from build123d import *

# Parameters (mm, degrees)
BOSS_EXTRUDE1_DEPTH  = 10
BOSS_EXTRUDE2_DEPTH  = 26.5
BOSS_EXTRUDE3_DEPTH  = 10
BOSS_EXTRUDE4_DEPTH  = 26.5
BOSS_EXTRUDE5_DEPTH  = 10
M2_CLEARANCE_HOLE1_D = 2.4


with BuildPart() as part:
    # Sketch2 → Boss-Extrude1 (new body)
    with BuildSketch(Plane.XY):
        Polygon((0, 0), (8, 0), (8, 1), (1, 1), (1, 6), (2.7, 6), (1.5, 7.2), (1, 7.2), (1, 9), (5.9, 9), (5.9, 10), (0, 10), align=None)
    extrude(amount=BOSS_EXTRUDE1_DEPTH)

    # Sketch6 → Boss-Extrude2 (add)
    with BuildSketch(Plane.XY.offset(10)):
        Polygon((0, 0), (5.9, 0), (5.9, 1), (1, 1), (1, 2.8), (2.7, 2.8), (2.7, 6), (1.5, 7.2), (1, 7.2), (1, 9), (5.9, 9), (5.9, 10), (0, 10), align=None)
    extrude(amount=BOSS_EXTRUDE2_DEPTH)

    # Sketch8 → Boss-Extrude3 (add)
    with BuildSketch(Plane.XY.offset(36.5)):
        Polygon((0, 0), (8, 0), (8, 1), (1, 1), (1, 6), (2.7, 6), (1.5, 7.2), (1, 7.2), (1, 9), (5.9, 9), (5.9, 10), (0, 10), align=None)
    extrude(amount=BOSS_EXTRUDE3_DEPTH)

    # Sketch9 → Boss-Extrude4 (add)
    with BuildSketch(Plane.XY.offset(46.5)):
        Polygon((0, 0), (5.9, 0), (5.9, 1), (1, 1), (1, 2.8), (2.7, 2.8), (2.7, 6), (1.5, 7.2), (1, 7.2), (1, 9), (5.9, 9), (5.9, 10), (0, 10), align=None)
    extrude(amount=BOSS_EXTRUDE4_DEPTH)

    # Sketch10 → Boss-Extrude5 (add)
    with BuildSketch(Plane.XY.offset(73)):
        Polygon((0, 0), (8, 0), (8, 1), (1, 1), (1, 6), (2.7, 6), (1.5, 7.2), (1, 7.2), (1, 9), (5.9, 9), (5.9, 10), (0, 10), align=None)
    extrude(amount=BOSS_EXTRUDE5_DEPTH)

    # M2 Clearance Hole1 (through all)
    with Locations(Plane(origin=(1, 0, 0), x_dir=(0, 0, -1), z_dir=(1, 0, 0))):
        with Locations((-2.8, 3.5), (-7.2, 3.5), (-39.3, 3.5), (-43.7, 3.5), (-75.8, 3.5), (-80.2, 3.5)):
            Hole(M2_CLEARANCE_HOLE1_D / 2)


solid = part.part
The model under review builds one solid part; all positions refer to its coordinate system, in mm. A direction names the side the tool comes from. Coordinates: 2 decimals unless noted, no trailing zeros. Order: outer loops, then holes, each group sorted by start corner. A loop starts at its lowest first (then second) coordinate and runs counter-clockwise, first axis right, second up. Notation, with made-up numbers: (47.5, 69) -> (100.5, 69) arc R12 cw to (100.5, 79) -> close; hole circle Ø3 at (69.5, -28.5). An arc over 180 degrees is marked (long way). Answer in a Markdown table with one row per item.
(1) Consider section A-A (x = 3.75). Write out the cut boundary in (y, z), plus the area to 3 significant figures.
Answers:
| item | result |
|---|---|
| outline | (0, 0) -> (1, 0) -> (1, 83) -> (0, 83) -> close; (9, 0) -> (10, 0) -> (10, 83) -> (9, 83) -> close |
| area | 166 mm² |
(2) Consider section B-B (z = 39.3). Write out the cut boundary in (x, y), plus the area to 3 significant figures.
Answers:
| item | result |
|---|---|
| outline | (0, 0) -> (8, 0) -> (8, 1) -> (1, 1) -> (1, 2.3) -> (0, 2.3) -> close; (0, 4.7) -> (1, 4.7) -> (1, 6) -> (2.7, 6) -> (1.5, 7.2) -> (1, 7.2) -> (1, 9) -> (5.9, 9) -> (5.9, 10) -> (0, 10) -> close |
| area | 20.8 mm² |
(3) Wall thickness on line 1 along Y through (x, z) = (1.5, 34); line 2 along Y through (x, z) = (0.6, 2.8); line 3 along Y through (x, z) = (4.75, 63): over which ranges is each line inside the solid? List them lowest first.
Answers:
| item | result |
|---|---|
| line 1 | 0 to 1, 2.8 to 7.2, 9 to 10 |
| line 2 | 0 to 2.3, 4.7 to 10 |
| line 3 | 0 to 1, 9 to 10 |
(4) Machinability: for faces 1 (the flat face through (0.7, 4.3, 83)), 2 (the flat face through (2, 4, 46.5)), 3 (the flat face through (2.7, 4, 60)), 4 (the flat face through (2, 6, 5)), which of the approach directions +Z, -Z, +X, -X, +Y, -Y give a long, thin tool a straight path to every point of the face, cutting with its end or side? Answer none if there is none.
Answers:
| item | result |
|---|---|
| face 1 | +Z, +X, -X, +Y, -Y |
| face 2 | +X |
| face 3 | +Z, -Z, +X |
| face 4 | -Z, +X |
(5) The part is to be moulded in two halves that separate along Z. For faces 5 (the flat face through (2, 6, 41)), 6 (the flat face through (2, 2.8, 23)), 7 (the flat face through (2, 4, 10)), say which applies: +Z half, -Z half, draft (parallel to the pull), parting line (faces both ways), or undercut.
Answers:
| item | result |
|---|---|
| face 5 | undercut |
| face 6 | draft |
| face 7 | -Z half |
(6) Insertion check: pin 1 (3 mm diameter, centred on y = 3.5, z = 39.3, fed in from +X); pin 2 (2 mm diameter, centred on y = 8.5, z = 61, fed in from +X); pin 3 (3.5 mm diameter, centred on y = 3.5, z = 26.5, fed in from +X). Each pin has a flat end and moves straight along its axis. Give the tip position at first contact, or say it passes through.
Answers:
| item | result |
|---|---|
| pin 1 | x = 1 |
| pin 2 | x = 5.9 |
| pin 3 | x = 2.7 |
(7) Consider section C-C (y = 3.5). State how many separate pieces and enclosed holes the cut face has, plus the area to 3 significant figures.
Answers:
| item | result |
|---|---|
| separate pieces | 7 |
| enclosed holes | 0 |
| area | 159 mm² |
(8) Consider section D-D (z = 22). Write out the cut boundary in (x, y).
Answers:
| item | result |
|---|---|
| outline | (0, 0) -> (5.9, 0) -> (5.9, 1) -> (1, 1) -> (1, 2.8) -> (2.7, 2.8) -> (2.7, 6) -> (1.5, 7.2) -> (1, 7.2) -> (1, 9) -> (5.9, 9) -> (5.9, 10) -> (0, 10) -> close |
